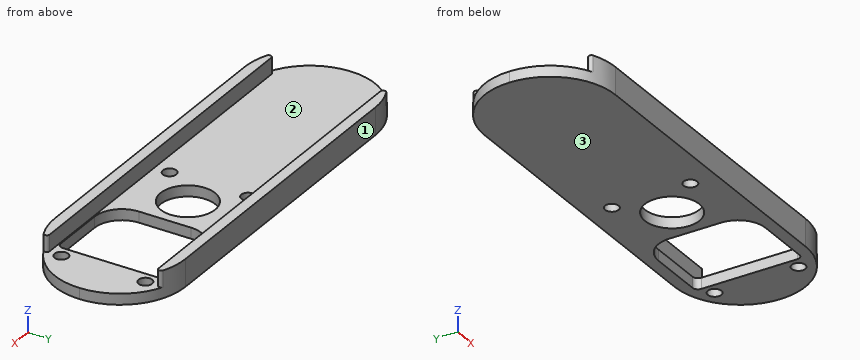
Autodesk Inventor part; units mm, degrees
ref_plane "YZ Plane" through (0, 0, 0) normal (1, 0, 0) x (0, 1, 0)
ref_plane "XZ Plane" through (0, 0, 0) normal (0, 1, 0) x (-1, 0, 0)
ref_plane "XY Plane" through (0, 0, 0) normal (0, 0, 1) x (1, 0, 0)
sketch "スケッチ1" plane through (0, 0, 0) normal (0, 0, 1) x (1, 0, 0)
  line L0 (-40, 12) -> (40, 12)
  line L1 (40, 12) -> (40, -12)
  line L2 (40, -12) -> (-40, -12)
  line L3 (-40, -12) -> (-40, 12)
  point P0 (0, 0)
  dimension "d0" = 80
  dimension "d1" = 24
  dimension "d2" = 12
  dimension "d3" = 40
extrude "押し出し1" add sketch "スケッチ1" along normal blind 5
sketch "スケッチ2" plane through (0, 0, 5) normal (0, 0, 1) x (1, 0, 0)
  line L0 (-0.8, 9.8) -> (35, 9.8)
  line L1 (35, 9.8) -> (35, -9.8)
  line L2 (35, -9.8) -> (-0.8, -9.8)
  line L3 (-0.8, -9.8) -> (-0.8, 9.8)
  line L4 (35, 9.8) -> (30.75, 9.8)
  line L5 (30.75, 9.8) -> (30.75, -9.8)
  line L6 (30.75, -9.8) -> (35, -9.8)
  line L7 (35, -9.8) -> (35, 9.8)
  line L8 (30.75, -9.8) -> (14.75, -9.8)
  line L9 (14.75, -9.8) -> (14.75, 9.8)
  line L10 (14.75, 9.8) -> (30.75, 9.8)
  line L11 (30.75, 9.8) -> (30.75, -9.8)
  circle A0 centre (8, 0) radius 5
  line L12 (35, 0) -> (-0.8, 0)
  circle A1 centre (1.8, 7.2) radius 1.25
  circle A2 centre (32.9, 7.7) radius 1.25
  circle A3 centre (1.8, -7.2) radius 1.25
  circle A4 centre (32.9, -7.7) radius 1.25
  line L13 (40, 12) -> (40, -12)
  point P0 (0, 0)
  dimension "d6" = 35.8
  dimension "d7" = 19.6
  dimension "d8" = 9.8
  dimension "d10" = 4.25
  dimension "d11" = 16
  dimension "d12" = 10
  dimension "d13" = 27
  dimension "d14" = 14.4
  dimension "d15" = 15.4
  dimension "d16" = 31.1
  dimension "d17" = 2.1
  dimension "d18" = 2.5
  dimension "d19" = 2.5
  dimension "d47" = 5
extrude "押し出し2" cut sketch "スケッチ2" against normal through all contours L0 L5 L12 L9 | L12 L5 L2 L9 | L12 A0 | A0 L12 | A1 | A2 | A3 | A4
fillet "フィレット1" radius 5 2 edges at (14.75, 9.8, 2.5) (14.75, -9.8, 2.5)
fillet "フィレット2" radius 1 2 edges at (30.75, 9.8, 2.5) (30.75, -9.8, 2.5)
sketch "スケッチ5" plane through (0, 0, 5) normal (0, 0, 1) x (1, 0, 0)
  line L0 (40, 12) -> (40, -12)
  line L1 (29.75, -9.8) -> (19.75, -9.8)
  arc A0 (14.75, -4.8) -> (19.75, -9.8) centre (19.75, -4.8) ccw
  line L2 (14.75, -4.8) -> (14.75, 4.8)
  arc A1 (19.75, 9.8) -> (14.75, 4.8) centre (19.75, 4.8) ccw
  line L3 (19.75, 9.8) -> (29.75, 9.8)
  arc A2 (30.75, 8.8) -> (29.75, 9.8) centre (29.75, 8.8) ccw
  line L4 (30.75, 8.8) -> (30.75, -8.8)
  arc A3 (29.75, -9.8) -> (30.75, -8.8) centre (29.75, -8.8) ccw
  circle A4 centre (32.9, -7.7) radius 1.25
  circle A5 centre (1.8, -7.2) radius 1.25
  circle A6 centre (32.9, 7.7) radius 1.25
  circle A7 centre (1.8, 7.2) radius 1.25
  circle A8 centre (8, 0) radius 5
  line L5 (40, 10) -> (-40, 10)
  line L6 (-40, 10) -> (-40, -10)
  line L7 (-40, -10) -> (40, -10)
  line L8 (40, -10) -> (40, 10)
  point P0 (-32.5, 14.4762)
  point P1 (-32.5, -14.4762)
  point P2 (0, 0)
  dimension "d41" = 20
  dimension "d42" = 10
  dimension "d49" = 41.8
extrude "押し出し4" cut sketch "スケッチ5" against normal blind 3
fillet "フィレット3" radius 12 4 edges at (40, -12, 2.5) (40, 12, 2.5) (-40, -12, 2.5) (-40, 12, 2.5)
fillet "フィレット4" radius 0.5 4 edges at (-34.6333, -10, 3.5) (-34.6333, 10, 3.5) (34.6333, 10, 3.5) (34.6333, -10, 3.5)
properties part number "JointC2"
Design review of the part built by this model. Coordinates are the model's own, in mm. Face numbers are marked on the shaded views. Round coordinates to 2 decimals unless told otherwise and drop trailing zeros. Order: outer loops, then holes, each group sorted by start corner. A loop starts at its lowest first (then second) coordinate and runs counter-clockwise, first axis right, second up.
1) Consider section C-C (y = -3.25). State the section outline as (x, z) points.
The answers:
outline: (-39.55, 0) - (4.2, 0) - (4.2, 2) - (-39.55, 2) - close; (11.8, 0) - (14.75, 0) - (14.75, 2) - (11.8, 2) - close; (30.75, 0) - (39.55, 0) - (39.55, 2) - (30.75, 2) - close
2) Clearance check with flat-ended pins moving along their axes: pin 1 Ø2 at (x, y) = (29, -2.5) entering from -Z (3 decimals); pin 2 Ø2 at (x, y) = (1.5, 0.5) entering from +Z; pin 3 Ø1.6 at (y, z) = (1.5, 1.5) entering from -X; pin 4 Ø3 at (y, z) = (7, 2) entering from +X. State where each tip first meets the part, or that it passes through.
The answers:
pin 1: passes through
pin 2: stops at z = 2
pin 3: stops at x = -39.98
pin 4: stops at x = 38.67
3) For L1, parallel to Y at x = 1.8, z = 1.1; L2, parallel to Y at x = 32.9, z = 0.5; L3, parallel to Y at x = 8, z = 4.3, list the stretches that pass through material, from the lowest coordinate up.
The answers:
L1: y = -12 to -8.45, -5.95 to 5.95, 8.45 to 12
L2: y = -10.95 to -8.95, -6.45 to 6.45, 8.95 to 10.95
L3: y = -12 to -10, 10 to 12
4) Consider section D-D (x = 6.5). State the section outline as (y, z) points.
The answers:
outline: (-12, 0) - (-4.77, 0) - (-4.77, 2) - (-10, 2) - (-10, 5) - (-12, 5) - close; (4.77, 0) - (12, 0) - (12, 5) - (10, 5) - (10, 2) - (4.77, 2) - close
5) Consider section B-B (x = -12). State the section outline as (y, z) points.
The answers:
outline: (-12, 0) - (12, 0) - (12, 5) - (10, 5) - (10, 2) - (-10, 2) - (-10, 5) - (-12, 5) - close
6) Draft analysis for pull direction Y (two halves, no side actions). For the marked faces 1, 2 and 3, state which applies: released by +Y, released by -Y, zero draft, split by the parting line, or undercut.
The answers:
face 1: released by +Y
face 2: undercut
face 3: zero draft
7) Consider section A-A (z = 3.3). State the section outline as (x, y) points.
The answers:
outline: (-32.89, -10.96) arc R12 ccw to (-28, -12) - (28, -12) arc R12 ccw to (32.89, -10.96) arc R0.5 ccw to (32.69, -10) - (-32.69, -10) arc R0.5 ccw to start; (-32.89, 10.96) arc R0.5 ccw to (-32.69, 10) - (32.69, 10) arc R0.5 ccw to (32.89, 10.96) arc R12 ccw to (28, 12) - (-28, 12) arc R12 ccw to start
